```python
from build123d import *

# Parameters (mm, degrees)
SKETCH_1_R          = 1.45
SKETCH_1_R_2        = 1.95
SKETCH_1_W          = 50
SKETCH_1_H          = 118
SKETCH_1_W_2        = 52
SKETCH_1_W_3        = 29.5
SKETCH_1_H_2        = 29.5
SKETCH_1_W_4        = 24
SKETCH_1_H_3        = 21.25
EXTRUDE_1_DEPTH     = 3
EXTRUDE_2_DEPTH     = 3
FILLET_1_R          = 3
FILLET_2_R          = 10
FILLET_3_R          = 10
SKETCH_3_W          = 13
SKETCH_3_H          = 10
SKETCH_3_R          = 1.45
EXTRUDE_3_DEPTH     = 3
FILLET_4_R          = 4
SKETCH_4_W          = 143.5
SKETCH_4_H          = 10
SKETCH_4_R          = 1.45
EXTRUDE_4_DEPTH     = 3
EXTRUDE_5_DEPTH     = 3
FILLET_5_R          = 3
CUT_EXTRUDE_1_DEPTH = 363.570338004
FILLET_6_R          = 2


with BuildPart() as part:
    # 草图1 → 凸台-拉伸1 (new body)
    with BuildSketch(Plane.XY):
        Polygon((0, 60), (-8, 60), (-33, 8), (-33, -7), (-87, -7), (-87, 8), (-70.75, 128.75), (0, 170), (8, 170), (8, 226), (140, 226), (140, 90), (35, 90), (8, 60), align=None)
        with Locations((-80, 0)):
            Circle(SKETCH_1_R, mode=Mode.SUBTRACT)
        with Locations((-40, 0)):
            Circle(SKETCH_1_R, mode=Mode.SUBTRACT)
        with Locations((0, 72.5)):
            Circle(SKETCH_1_R, mode=Mode.SUBTRACT)
        with Locations((0, 92.5)):
            Circle(SKETCH_1_R, mode=Mode.SUBTRACT)
        with Locations((0, 132.5)):
            Circle(SKETCH_1_R, mode=Mode.SUBTRACT)
        with Locations((0, 152.5)):
            Circle(SKETCH_1_R, mode=Mode.SUBTRACT)
        with Locations((-58.75, 128.75)):
            Circle(SKETCH_1_R, mode=Mode.SUBTRACT)
        with Locations((-21.25, 128.75)):
            Circle(SKETCH_1_R, mode=Mode.SUBTRACT)
        with Locations((-21.25, 91.25)):
            Circle(SKETCH_1_R, mode=Mode.SUBTRACT)
        with Locations((-58.75, 91.25)):
            Circle(SKETCH_1_R, mode=Mode.SUBTRACT)
        with Locations((75, 206)):
            Circle(SKETCH_1_R_2, mode=Mode.SUBTRACT)
        with Locations((75, 110)):
            Circle(SKETCH_1_R_2, mode=Mode.SUBTRACT)
        with Locations((45, 159)):
            Rectangle(SKETCH_1_W, SKETCH_1_H, mode=Mode.SUBTRACT)
        with Locations((106, 159)):
            Rectangle(SKETCH_1_W_2, SKETCH_1_H, mode=Mode.SUBTRACT)
        Polygon((-15, 77.75059269), (-48.533938793, 8), (-80.945912041, 8), (-70.415373738, 86.25), (-15, 86.25), align=None, mode=Mode.SUBTRACT)
        Polygon((-52.247328604, 133.75), (-6, 160.713990175), (-6, 133.75), align=None, mode=Mode.SUBTRACT)
        with Locations((-40, 110)):
            Rectangle(SKETCH_1_W_3, SKETCH_1_H_2, mode=Mode.SUBTRACT)
        with Locations((0, 113.125)):
            Rectangle(SKETCH_1_W_4, SKETCH_1_H_3, mode=Mode.SUBTRACT)
    extrude(amount=EXTRUDE_1_DEPTH)

    # 草图2 → 凸台-拉伸2 (add)
    with BuildSketch(Plane.XY):
        Polygon((70, 218), (26.39653383, 100), (20, 100), (63.60346617, 218), align=None)
        Polygon((80, 100), (123.60346617, 218), (132, 218), (88.39653383, 100), align=None)
        Polygon((-48.533938793, 8), (-70.415373738, 86.25), (-65.223563587, 86.25), (-45.251391654, 14.82769805), align=None)
    extrude(amount=EXTRUDE_2_DEPTH)

    # 圆角1
    fillet_1_edges = [part.edges().sort_by_distance(p)[0] for p in [
        (-15, 77.75059269, 1.5),
        (-15, 86.25, 1.5),
        (-70.415373738, 86.25, 1.5),
        (-80.945912041, 8, 1.5),
        (-48.533938793, 8, 1.5),
        (-25.25, 95.25, 1.5),
        (-25.25, 124.75, 1.5),
        (-54.75, 124.75, 1.5),
        (-54.75, 95.25, 1.5),
        (-52.247328604, 133.75, 1.5),
        (-6, 133.75, 1.5),
        (-6, 160.713990175, 1.5),
        (12, 102.5, 1.5),
        (12, 123.75, 1.5),
        (-12, 123.75, 1.5),
        (-12, 102.5, 1.5),
        (-45.251391654, 14.82769805, 1.5),
        (-65.223563587, 86.25, 1.5),
        (88.39653383, 100, 1.5),
        (123.60346617, 218, 1.5),
        (63.60346617, 218, 1.5),
        (26.39653383, 100, 1.5),
        (70, 100, 1.5),
        (70, 218, 1.5),
        (20, 218, 1.5),
        (20, 100, 1.5),
        (132, 100, 1.5),
        (132, 218, 1.5),
        (80, 218, 1.5),
        (80, 100, 1.5),
    ]]
    fillet(fillet_1_edges, radius=FILLET_1_R)

    # 圆角2
    # the kernel refuses this fillet: 10 mm, written as the material it adds along each edge
    with BuildSketch(Plane(origin=(8, 170, 0), x_dir=(-1, 0, 0), z_dir=(0, 0, 1))) as fillet_2_piece_1:
        with BuildLine():
            CenterArc((10, -9.797958971), FILLET_2_R, 101.536959033, 78.463040967)
            Line((0, -9.797958971), (-0.2, -9.797958971))
            Line((-0.2, -9.797958971), (-0.2, 0))
            Line((-0.2, 0), (0, 0.2))
            ThreePointArc((0, 0.2), (4, 0.2), (7.96, 0.195959179))
            Line((7.96, 0.195959179), (8, 0))
        make_face()
    extrude(amount=3)

    # 圆角3
    fillet_3_edges = [part.edges().sort_by_distance(p)[0] for p in [
        (-8, 60, 1.5),
        (-33, 8, 1.5),
        (-33, -7, 1.5),
        (-87, -7, 1.5),
        (-87, 8, 1.5),
        (-70.75, 128.75, 1.5),
        (0, 170, 1.5),
        (8, 226, 1.5),
        (140, 226, 1.5),
        (140, 90, 1.5),
        (35, 90, 1.5),
        (8, 60, 1.5),
    ]]
    fillet(fillet_3_edges, radius=FILLET_3_R)

    # 草图3 → 凸台-拉伸3 (add)
    with BuildSketch(Plane.XY):
        with Locations((1.5, 192.5)):
            Rectangle(SKETCH_3_W, SKETCH_3_H)
        with Locations((0, 192.5)):
            Circle(SKETCH_3_R, mode=Mode.SUBTRACT)
    extrude(amount=EXTRUDE_3_DEPTH)

    # 圆角4
    fillet_4_edges = [part.edges().sort_by_distance(p)[0] for p in [
        (-5, 187.5, 1.5),
        (-5, 197.5, 1.5),
        (8, 197.5, 1.5),
        (8, 187.5, 1.5),
    ]]
    fillet(fillet_4_edges, radius=FILLET_4_R)

    # 草图4 → 凸台-拉伸4 (add)
    with BuildSketch(Plane.XY):
        with Locations((211.75, 147.5)):
            Rectangle(SKETCH_4_W, SKETCH_4_H)
        with Locations((277.5, 147.5)):
            Circle(SKETCH_4_R, mode=Mode.SUBTRACT)
    extrude(amount=EXTRUDE_4_DEPTH)

    # 草图5 → 凸台-拉伸5 (add)
    with BuildSketch(Plane.XY):
        Polygon((283.5, 152.5), (140, 176.5), (140, 170.5), (247.625, 152.5), align=None)
    extrude(amount=EXTRUDE_5_DEPTH)

    # 圆角5
    fillet_5_edges = [part.edges().sort_by_distance(p)[0] for p in [
        (283.5, 152.5, 1.5),
        (283.5, 142.5, 1.5),
        (140, 142.5, 1.5),
        (140, 152.5, 1.5),
        (247.625, 152.5, 1.5),
        (140, 176.5, 1.5),
        (140, 170.5, 1.5),
    ]]
    fillet(fillet_5_edges, radius=FILLET_5_R)

    # 草图6 → 切除-拉伸1 (cut, through all)
    with BuildSketch(Plane.XY.offset(3)):
        Polygon((8, 90), (8, 68.969082698), (26.927825572, 90), align=None)
    extrude(amount=-CUT_EXTRUDE_1_DEPTH, mode=Mode.SUBTRACT)

    # 圆角6
    fillet_6_edges = [part.edges().sort_by_distance(p)[0] for p in [
        (8, 90, 1.5),
        (26.927825572, 90, 1.5),
        (8, 68.969082698, 1.5),
    ]]
    fillet(fillet_6_edges, radius=FILLET_6_R)


solid = part.part
```
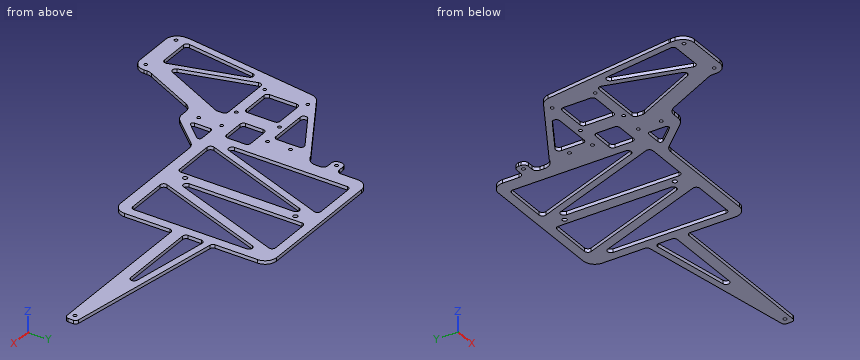
The listing builds one solid part. Answer for the finished solid, in the listing's coordinates (mm). Give positions to 0.01 mm unless a question says otherwise; leave off trailing zeros. Write each loop counter-clockwise with the first axis right and the second up, starting at its lowest first coordinate (ties: lowest second). Pieces come first, ordered by that corner, then holes. Notation, with made-up numbers: (3, 39.5) -> (30, 39.5) arc R19 ccw to (30, 44.5) -> close; hole circle Ø8 at (-0.75, -30). An arc over 180 degrees is marked (long way). Write item = value, one per line. Start each with the question number.
1) The part is cut by section A-A, the plane x = 102.5. Determine the outline of the cut face in (y, z), and give its area (3 significant figures).
2) Straight lines are drawn through the part: line 1 along Y through (x, z) = (75, 1.7); line 2 along X through (y, z) = (91.25, 0.85); line 3 along X through (y, z) = (186, 1.8). For each, find the intervals that lie inside material, in ascending order.
3) The part is cut by section B-B, the plane z = 0.7. Count the separate pieces of the cut face and the enclosed holes in it, and give its area (3 significant figures).
4) The part is cut by section C-C, the plane x = 45.5. Determine the outline of the cut face in (y, z), and give its area (3 significant figures).
5) Each of these flat-tipped pins is pushed along its axis until it touches: pin 1 (2.5 mm diameter, centred on x = -80, y = 0, fed in from +Z); pin 2 (1 mm diameter, centred on x = 180.5, z = 0.5, fed in from -Y); pin 3 (1.5 mm diameter, centred on y = 119, z = 2, fed in from +X); pin 4 (0.9 mm diameter, centred on x = -4, z = 1, fed in from +Y). Where does it stop, or does it pass through?
Solutions:
q1.outline = (90, 0) -> (100, 0) -> (100, 3) -> (90, 3) -> close; (138.17, 0) -> (160.89, 0) -> (160.89, 3) -> (138.17, 3) -> close; (218, 0) -> (226, 0) -> (226, 3) -> (218, 3) -> close
q1.area = 122 mm²
q2.line_1 = 90 to 108.05, 111.95 to 204.05, 207.95 to 226
q2.line_2 = -75.8 to -60.2, -57.3 to -22.7, -19.8 to -0.73, 0.73 to 134.84
q2.line_3 = 7.12 to 20, 51.78 to 58.18, 70 to 80, 111.78 to 120.18, 132 to 140
q3.separate_pieces = 1
q3.enclosed_holes = 25
q3.area = 16,800 mm²
q4.outline = (90, 0) -> (100, 0) -> (100, 3) -> (90, 3) -> close; (151.7, 0) -> (169.01, 0) -> (169.01, 3) -> (151.7, 3) -> close; (218, 0) -> (226, 0) -> (226, 3) -> (218, 3) -> close
q4.area = 106 mm²
q5.pin_1 = through
q5.pin_2 = 142.5
q5.pin_3 = 140
q5.pin_4 = 196.58
